```python
from build123d import *

# Parameters (mm, degrees)
SKETCH2_R           = 10
BOSS_EXTRUDE1_DEPTH = 63
SKETCH3_R           = 12.5
BOSS_EXTRUDE2_DEPTH = 60
SKETCH5_R           = 5.9
CUT_EXTRUDE1_DEPTH  = 40
SKETCH6_R           = 2.5
CUT_EXTRUDE2_DEPTH  = 55
CIRPATTERN1_COUNT   = 3
SKETCH8_R           = 9
BOSS_EXTRUDE3_DEPTH = 77
SKETCH9_W           = 3.883559786
SKETCH9_H           = 4
CUT_EXTRUDE3_DEPTH  = 50


with BuildPart() as part:
    # Sketch2 → Boss-Extrude1 (new body)
    with BuildSketch(Plane(origin=(0, 0, 0), x_dir=(0, 0, -1), z_dir=(1, 0, 0))):
        Circle(SKETCH2_R)
    extrude(amount=BOSS_EXTRUDE1_DEPTH)

    # Sketch3 → Boss-Extrude2 (add)
    with BuildSketch(Plane(origin=(63, 0, 0), x_dir=(0, 0, -1), z_dir=(1, 0, 0))):
        Circle(SKETCH3_R)
    extrude(amount=BOSS_EXTRUDE2_DEPTH)

    # Sketch5 → Cut-Extrude1 (cut)
    with BuildSketch(Plane(origin=(123, 0, 0), x_dir=(0, 0, -1), z_dir=(1, 0, 0))):
        Circle(SKETCH5_R)
    extrude(amount=-CUT_EXTRUDE1_DEPTH, mode=Mode.SUBTRACT)

    # Sketch6 → Cut-Extrude2 (cut)
    with BuildSketch(Plane(origin=(0, 0, 0), x_dir=(1, 0, 0), z_dir=(0, 1, 0))):
        with Locations(Location((93, 0, 0), (0, 0, 270))):
            Circle(SKETCH6_R)
        with Locations(Location((111, 0, 0), (0, 0, 270))):
            Circle(SKETCH6_R)
    cut_extrude2 = extrude(amount=-CUT_EXTRUDE2_DEPTH, mode=Mode.SUBTRACT)

    # CirPattern1: Cut-Extrude2 ×3 about axis
    cirpattern1_axis = Axis((123, 0, 0), (1, 0, 0))
    for i in range(1, CIRPATTERN1_COUNT):
        add(cut_extrude2.rotate(cirpattern1_axis, i * 360 / CIRPATTERN1_COUNT), mode=Mode.SUBTRACT)

    # Sketch8 → Boss-Extrude3 (add)
    with BuildSketch(Plane.ZY):
        with Locations(Location((0, 0, 0), (0, 0, 180))):
            Circle(SKETCH8_R)
    extrude(amount=BOSS_EXTRUDE3_DEPTH)

    # Sketch9 → Cut-Extrude3 (cut)
    with BuildSketch(Plane.ZY.offset(77)):
        with Locations((8.441779893, 0)):
            Rectangle(SKETCH9_W, SKETCH9_H)
    extrude(amount=-CUT_EXTRUDE3_DEPTH, mode=Mode.SUBTRACT)


solid = part.part
```
Geometry: final body of the model. Coordinates: model frame, mm. A direction names the side the tool comes from. Give positions to 0.01 mm unless a question says otherwise; leave off trailing zeros. Write each loop counter-clockwise with the first axis right and the second up, starting at its lowest first coordinate (ties: lowest second). Pieces come first, ordered by that corner, then holes.
1. Section query B-B, the plane x = 93. Return loops of the section in (y, z), then the cut area to 3 significant figures.
2. Line query: probe 1 along X at (y, z) = (-9.5, 0); probe 2 along X at (y, z) = (-8.75, 0); probe 3 along Z at (x, y) = (-59.5, 0.25). Output: solid intervals per line, ascending.
3. Section query A-A, the plane z = 0. Return loops of the section in (x, y), then the cut area to 3 significant figures.
4. Section query C-C, the plane x = -15. Return loops of the section in (y, z), then the cut area to 3 significant figures.
5. Reachability of faces 1 (the cylindrical face through (92.58, 3.755, -11.923)), 2 (the flat face through (-52, 0, 6.5)), 3 (the flat face through (83, 0, 0)), 4 (the cylindrical face through (31.06, -9.76, 2.17)), 5 (the cylindrical face through (93.1, -8.9, -2.5)) from +Z, -Z, +X, -X, +Y, -Y: full face, straight path, thin tool, end or side. Return the list, or none.
6. Draft query along Y for faces 6 (the cylindrical face through (-37.961, -2.703, -8.584)), 7 (the cylindrical face through (103.28, -3.59, 4.68)), 8 (the cylindrical face through (111.1, -8.9, -2.5)), 9 (the cylindrical face through (111.11, 2.275, 8.935)). Return one class per face: released by +Y, released by -Y, zero draft, split by the parting line, or undercut.
7. Pin query (flat end, axial travel): P1, Ø6, axis at x = 28, z = -4.5, coming from the -Y side; P2, Ø0.7, axis at x = -41.5, z = 8, coming from the -Y side; P3, Ø7, axis at y = 0, z = 0, coming from the +X side. Return the tip coordinate at first contact, or that it passes through.
Computed:
1. outline: (-12.25, -2.5) arc R12.5 ccw to (3.96, -11.86) - (0.51, -5.88) arc R5.9 cw to (-5.34, -2.5) - close; (-12.25, 2.5) - (-5.34, 2.5) arc R5.9 cw to (0.51, 5.88) - (3.96, 11.86) arc R12.5 ccw to start; (4.84, -3.38) - (8.29, -9.36) arc R12.5 ccw to (8.29, 9.36) - (4.84, 3.38) arc R5.9 cw to start
1. area: 281 mm2
2. probe 1: x = 0 to 90.5, 95.5 to 108.5, 113.5 to 123
2. probe 2: x = -77 to 90.5, 95.5 to 108.5, 113.5 to 123
2. probe 3: z = -9 to 6.5
3. outline: (-77, -9) - (0, -9) - (0, -10) - (63, -10) - (63, -12.5) - (90.5, -12.5) - (90.5, -5.9) - (83, -5.9) - (83, 5.9) - (123, 5.9) - (123, 12.5) - (63, 12.5) - (63, 10) - (0, 10) - (0, 9) - (-77, 9) - close; (95.5, -12.5) - (108.5, -12.5) - (108.5, -5.9) - (95.5, -5.9) - close; (113.5, -12.5) - (123, -12.5) - (123, -5.9) - (113.5, -5.9) - close
3. area: 3,610 mm2
4. outline: circle Ø18 at (0, 0)
4. area: 254 mm2
5. face 1: +X, -X
5. face 2: +Z, -X
5. face 3: +X
5. face 4: -X
5. face 5: -Y
6. face 6: split by the parting line
6. face 7: undercut
6. face 8: zero draft
6. face 9: undercut
7. P1: stops at y = -9.89
7. P2: stops at y = -4.74
7. P3: stops at x = 83
